Model file for the job. Use its own axes, mm. A direction names the side the tool comes from. Round coordinates to 2 decimals unless told otherwise and drop trailing zeros. Order: outer loops, then holes, each group sorted by start corner. A loop starts at its lowest first (then second) coordinate and runs counter-clockwise, first axis right, second up. Notation, with made-up numbers: (39, 51.5) - (70, 51.5) arc R24 cw to (70, 74.5) - close; hole circle Ø8 at (-18.5, 83). An arc over 180 degrees is marked (long way). Write item = value, one per line. Start each with the question number.
Autodesk Inventor part; units mm, degrees
ref_plane "Work Plane7" through (-19.4482, 115.8757, 12.2593) normal (0, 0, 1) x (1, 0, 0)
ref_plane "YZ Plane" through (0, 0, 0) normal (1, 0, 0) x (0, 1, 0)
ref_plane "XZ Plane" through (0, 0, 0) normal (0, 1, 0) x (-1, 0, 0)
ref_plane "Work Plane1" through (-0.2955, 151.1757, 22.2593) normal (-1, 0, 0) x (0, -1, 0)
sketch "Sketch1" plane through (-0.2955, 151.1757, 22.2593) normal (-1, 0, 0) x (0, -1, 0)
  arc A0 (59.8, 2) -> (63.9581, 11.1) centre (59.8, 7.5) ccw
  circle A1 centre (59.8, 7.5) radius 1.4305
  point P0 (151.1757, -22.2593)
extrude "Extrusion1" add sketch "Sketch1" along normal blind 30
ref_plane "Work Plane2" through (-18.4955, 91.3757, 29.7593) normal (-1, 0, 0) x (0, -1, 0)
ref_plane "Work Plane4" through (-30.2955, 91.3757, 29.7593) normal (0, -1, 0) x (1, 0, 0)
ref_plane "Work Plane3" through (-0.2955, 73.8757, 22.2593) normal (0, -1, 0) x (1, 0, 0)
sketch "Sketch2" plane through (-30.2955, 91.3757, 29.7593) normal (0, -1, 0) x (1, 0, 0)
  line L0 (0, 1.4305) -> (0, -1.4305)
  line L1 (30, -1.4305) -> (30, 1.4305)
  circle A0 centre (11.8, 0) radius 1.4305
  line L2 (30, -1.4305) -> (0, -1.4305)
  line L3 (26.8, 6.34) -> (26.8, -6.34)
  point P0 (30.2955, -29.7593)
  dimension "d2" = 15
extrude "Extrusion2" add sketch "Sketch2" against normal blind 50
ref_plane "Work Plane6" through (-18.4955, 141.3757, 29.7593) normal (0, 0, 1) x (1, 0, 0)
ref_plane "Work Plane5" through (74.7045, 112.5257, 35.3593) normal (0, 0, 1) x (1, 0, 0)
sketch "Sketch3" plane through (-18.4955, 141.3757, 29.7593) normal (0, 0, 1) x (1, 0, 0)
  line L0 (1.4305, 0) -> (-1.4305, 0)
  circle A0 centre (0, 0) radius 1.4305
  line L1 (1.4305, -48.5695) -> (1.4305, 0)
  point P0 (18.4955, -141.3757)
ref_plane "Work Plane7" through (-19.4482, 115.8757, 12.2593) normal (0, 0, 1) x (1, 0, 0)
extrude "Extrusion3" add sketch "Sketch3" against normal up to surface (17.5 mm away)
ref_plane "Work Plane10" through (-18.4955, 141.3757, 29.7593) normal (0, -0.7071, 0.7071) x (-1, 0, 0)
ref_plane "Work Plane9" through (-18.4955, 141.3757, 12.2593) normal (0, -1, 0) x (1, 0, 0)
ref_plane "Work Plane8" through (-57.7234, 76.1875, 20.0898) normal (0, -1, 0) x (1, 0, 0)
properties part number "00_Lightpath"
Item 1: Mould opens along Y. For faces 5 (the face through (-17.13, 116.03, 30.19)), 6 (the face through (-30.296, 91, 30)), 7 (the face through (-19, 141.376, 30)) say: +Y half, -Y half, draft (parallel to the pull), parting line (faces both ways), or undercut.
Item 2: Which spindle directions (+Z, -Z, +X, -X, +Y, -Y) get a long thin tool onto all of the face, cutting with end or side? Do faces 1 (the face through (-15.09, 90.01, 29.33)), 2 (the face through (-0.296, 91, 30)), 3 (the face through (-18.682, 142.794, 21.132)), 4 (the face through (-19, 142, 29.759)). Say none if no direction does.
Item 3: Probe L1, parallel to Y at x = -18.5, z = 23.5; L2, parallel to Z at x = -19.75, y = 106; L3, parallel to Y at x = -17.75, z = 30.75. List the from-to ranges inside material, lowest first.
Item 4: Saw through at A-A, the plane x = -17.75. Give the cut face in (y, z).
Item 5: Drop flat-ended pins along their axis: pin 1 (1.1 mm diameter, centred on x = -19, z = 30.5, fed in from +Y); pin 2 (1.5 mm diameter, centred on x = -17.5, y = 126.5, fed in from +Z); pin 3 (0.7 mm diameter, centred on x = -19, y = 142, fed in from +Z). Give the stop position or say it passes through.
Item 6: Saw through at C-C, the plane y = 103.5. Give the cut face in (x, z) (1 decimal).
Item 7: Saw through at B-B, the plane z = 24.5. Give the cut face in (x, y) (1 decimal).
Check sheet entries:
q1.face_5 = undercut
q1.face_6 = draft
q1.face_7 = +Y half
q2.face_1 = none
q2.face_2 = +Z, -Z, +X, +Y, -Y
q2.face_3 = -Z
q2.face_4 = +Z, +X, -X, +Y
q3.L1 = 139.95 to 142.81
q3.L2 = 29.07 to 30.45
q3.L3 = 90.34 to 141.38
q4.outline = (92.12, 28.54) - (140.15, 28.54) - (140.15, 12.26) - (142.6, 12.26) - (142.6, 29.76) - (141.38, 29.76) - (141.38, 30.98) - (92.12, 30.98) arc R1.43 ccw (long way) to start
q5.pin_1 = 141.38
q5.pin_2 = 31.17
q5.pin_3 = 29.76
q6.outline = circle Ø2.9 at (-18.5, 29.8)
q7.outline = circle Ø2.9 at (-18.5, 141.4)
